Build history of the part. All positions in model axes, mm. Round coordinates to 2 decimals unless told otherwise and drop trailing zeros. Loops run counter-clockwise (first coordinate to the right, second up) from the corner with the lowest first, then second, coordinate; pieces in that order, holes last. Notation, with made-up numbers: (-33.75, 16) - (-29.75, 16) arc R22 cw to (-29.75, 49) - close; hole circle Ø2 at (-31, -21). An arc over 180 degrees is marked (long way). Answer as CSV lines item,"result". Start each with the question number.
```python
from build123d import *

# Parameters (mm, degrees)
SKETCH_R     = 12
PAD_DEPTH    = 317
PAD001_DEPTH = 5
SKETCH004_R  = 12.2
PAD003_DEPTH = 17
PAD004_DEPTH = 36
SKETCH006_R  = 5
POCKET_DEPTH = 28.001


with BuildPart() as part:
    # Sketch → Pad (new body)
    with BuildSketch(Plane.XY):
        Circle(SKETCH_R)
    extrude(amount=PAD_DEPTH)

    # Sketch001 → Pad001 (join)
    with BuildSketch(Plane.XY):
        with BuildLine():
            ThreePointArc((-4.482187, 14), (-14.7, 0), (-4.482187, -14))
            Line((-4.482187, -14), (4.482187, -14))
            ThreePointArc((4.482187, -14), (14.7, 0), (4.482187, 14))
            Line((-4.482187, 14), (4.482187, 14))
        make_face()
    extrude(amount=-PAD001_DEPTH)

    # Sketch004 (on Face2 of Pad) → Pad003 (join)
    with BuildSketch(Plane(origin=(0, 0, 0), x_dir=(1, 0, 0), z_dir=(0, 0, -1))):
        Circle(SKETCH004_R)
    extrude(amount=-PAD003_DEPTH)

    # Sketch005 (on Face5 of Pad003) → Pad004 (join)
    with BuildSketch(Plane(origin=(0, 0, -5), x_dir=(1, 0, 0), z_dir=(0, 0, -1))):
        with BuildLine():
            ThreePointArc((-4.482187, 14), (-10.199256, 10.586084), (-13.823531, 5))
            Line((-13.823531, 5), (13.823531, 5))
            ThreePointArc((13.823531, 5), (10.199256, 10.586084), (4.482187, 14))
            Line((-4.482187, 14), (4.482187, 14))
        make_face()
        with BuildLine():
            Line((-13.823531, -5), (13.823531, -5))
            ThreePointArc((4.482187, -14), (10.199256, -10.586084), (13.823531, -5))
            Line((4.482187, -14), (-4.482187, -14))
            ThreePointArc((-13.823531, -5), (-10.199256, -10.586084), (-4.482187, -14))
        make_face()
    extrude(amount=PAD004_DEPTH)

    # Sketch006 (on Face9 of Pad004) → Pocket (cut, through all)
    with BuildSketch(Plane(origin=(0, 14, 0), x_dir=(-1, 0, 0), z_dir=(0, 1, 0))):
        with Locations((0, -21.5)):
            Circle(SKETCH006_R)
        with BuildLine():
            ThreePointArc((-18.5, -21.5), (0, -40), (18.5, -21.5))
            Line((18.5, -21.5), (18.5, -43))
            Line((-18.5, -43), (18.5, -43))
            Line((-18.5, -21.5), (-18.5, -43))
        make_face()
    extrude(amount=-POCKET_DEPTH, mode=Mode.SUBTRACT)


solid = part.part
```
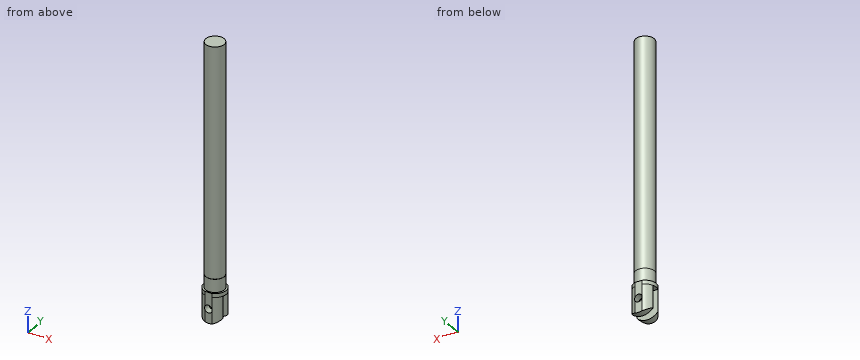
Q1. Band-saw the part on C-C, the plane z = 135.5. List the corners of the cut face in (x, y), then the cut area to 3 significant figures.
Q2. Band-saw the part on B-B, the plane y = 0. List the corners of the cut face in (x, z).
Q3. Band-saw the part on A-A, the plane x = 0. List the corners of the cut face in (y, z).
Q4. Pin check, flat tips, straight feed: pin 1 Ø10 at (y, z) = (8.5, 19.5) entering from +X; pin 2 Ø11.5 at (x, z) = (0, -21.5) entering from -Y; pin 3 Ø8 at (x, y) = (-11.5, 9.5) entering from -Z; pin 4 Ø6 at (y, z) = (-2, 116) entering from +X. Stop position of each tip, or through.
Q5. Wall check: probe 1 along X at (y, z) = (8.5, -21.5); probe 2 along Z at (x, y) = (0, 7.75); probe 3 along X at (y, z) = (8.75, -21.5). Give the ranges that are in metal, low to high. Write a range as [from, to].
Reported:
1,outline,"circle Ø24 at (0, 0)"
1,area,"452 mm2"
2,outline,"(-14.7, -5) - (14.7, -5) - (14.7, 0) - (12.2, 0) - (12.2, 17) - (12, 17) - (12, 317) - (-12, 317) - (-12, 17) - (-12.2, 17) - (-12.2, 0) - (-14.7, 0) - close"
3,outline,"(-14, -40) - (-5, -40) - (-5, -26.5) - (-14, -26.5) - close; (-14, -16.5) - (-5, -16.5) - (-5, -5) - (5, -5) - (5, -16.5) - (14, -16.5) - (14, 0) - (12.2, 0) - (12.2, 17) - (12, 17) - (12, 317) - (-12, 317) - (-12, 17) - (-12.2, 17) - (-12.2, 0) - (-14, 0) - close; (5, -40) - (14, -40) - (14, -26.5) - (5, -26.5) - close"
4,pin 1,"stops at x = 11.48"
4,pin 2,"stops at y = -14"
4,pin 3,"stops at z = -38.41"
4,pin 4,"stops at x = 12"
5,probe 1,"x = [-11.99, -5], [5, 11.99]"
5,probe 2,"z = [-40, -26.5], [-16.5, 317]"
5,probe 3,"x = [-11.81, -5], [5, 11.81]"
